Design review of the part built by this model. Coordinates are the model's own, in mm. A direction names the side the tool comes from. Coordinates: 2 decimals unless noted, no trailing zeros. Order: outer loops, then holes, each group sorted by start corner. A loop starts at its lowest first (then second) coordinate and runs counter-clockwise, first axis right, second up.
from build123d import *

# Parameters (mm, degrees)
CROQUIS1_R              = 25
SALIENTE_EXTRUIR1_DEPTH = 13
CROQUIS2_R              = 11.5
SALIENTE_EXTRUIR2_DEPTH = 2
CROQUIS3_R              = 9.5
CORTAR_EXTRUIR1_DEPTH   = 10
CROQUIS4_R              = 6.5
CORTAR_EXTRUIR2_DEPTH   = 37.742346142


with BuildPart() as part:
    # Croquis1 → Saliente-Extruir1 (new body)
    with BuildSketch(Plane.XY):
        Circle(CROQUIS1_R)
    extrude(amount=-SALIENTE_EXTRUIR1_DEPTH)

    # Croquis2 → Saliente-Extruir2 (add)
    with BuildSketch(Plane.XY):
        Circle(CROQUIS2_R)
    extrude(amount=SALIENTE_EXTRUIR2_DEPTH)

    # Croquis3 → Cortar-Extruir1 (cut)
    with BuildSketch(Plane.XY.offset(2)):
        Circle(CROQUIS3_R)
    extrude(amount=-CORTAR_EXTRUIR1_DEPTH, mode=Mode.SUBTRACT)

    # Croquis4 → Cortar-Extruir2 (cut, through all)
    with BuildSketch(Plane.XY.offset(-8)):
        Circle(CROQUIS4_R)
    extrude(amount=-CORTAR_EXTRUIR2_DEPTH, mode=Mode.SUBTRACT)


solid = part.part
1. For faces 5 (the cylindrical face through (23.846, 7.509, -6.409)), 6 (the flat face through (5, -11, 0)), list the 3-axis set-ups (+Z, -Z, +X, -X, +Y, -Y) from which the entire face can be reached by the end or side of a thin tool; tool diameter is ignored.
2. Add section A-A (x = 0). Give the boundary of the cut face in (y, z), and give its area (3 significant figures).
3. Insertion check: pin 1 (8 mm diameter, centred on x = 0, y = 0, fed in from +Z); pin 2 (1 mm diameter, centred on x = 9.5, z = -9.5, fed in from -Y); pin 3 (4 mm diameter, centred on y = 20, z = -7, fed in from -X). Each pin has a flat end and moves straight along its axis. Give the tip position at first contact, or say it passes through.
4. Mouldability with a two-part tool opening along Y and no side actions: class faces 1 (the flat face through (-4, 9, 2)), 2 (the cylindrical face through (-5.158, -3.955, -10.465)), 3 (the cylindrical face through (4.38, -8.43, -2.93)), 4 (the cylindrical face through (-1.5, 11.4, 1)) as pulls with the +Y half, pulls with the -Y half, needs draft (parallel to the pull), parting line crosses it, or undercut.
5. Add section C-C (z = -1.5). Give the boundary of the cut face in (x, y).
6. To check wall thickness, follow line 1 (Y direction, x = 0, z = -9.55); line 2 (Y direction, x = 0, z = -5.75); line 3 (Z direction, x = 3, y = 18). State the ranges of each line that lie inside material, in increasing order.
7. Add section D-D (y = 8). Give the boundary of the cut face in (x, z), and give its area (3 significant figures).
Solution:
1. face 5: +Z, -Z
1. face 6: +Z
2. outline: (-25, -13) - (-6.5, -13) - (-6.5, -8) - (-9.5, -8) - (-9.5, 2) - (-11.5, 2) - (-11.5, 0) - (-25, 0) - close; (6.5, -13) - (25, -13) - (25, 0) - (11.5, 0) - (11.5, 2) - (9.5, 2) - (9.5, -8) - (6.5, -8) - close
2. area: 441 mm2
3. pin 1: passes through
3. pin 2: stops at y = -23.32
3. pin 3: stops at x = -17.35
4. face 1: needs draft
4. face 2: undercut
4. face 3: undercut
4. face 4: parting line crosses it
5. outline: circle Ø50 at (0, 0); hole circle Ø19 at (0, 0)
6. line 1: y = -25 to -6.5, 6.5 to 25
6. line 2: y = -25 to -9.5, 9.5 to 25
6. line 3: z = -13 to 0
7. outline: (-23.69, -13) - (23.69, -13) - (23.69, 0) - (8.26, 0) - (8.26, 2) - (5.12, 2) - (5.12, -8) - (-5.12, -8) - (-5.12, 2) - (-8.26, 2) - (-8.26, 0) - (-23.69, 0) - close
7. area: 546 mm2
